```python
from build123d import *

# Parameters (mm, degrees)
BOSS_EXTRUDE1_DEPTH           = 10
BOSS_EXTRUDE1_DEPTH_BACK      = 10
SKETCH1_W                     = 11
SKETCH1_H                     = 11
SKETCH3_R                     = 1.65
M4_THREADED_3_3_MM_THRU_DEPTH = 38.199596772
CUT_EXTRUDE1_DEPTH            = 4.3
CUT_EXTRUDE1_DEPTH_BACK       = 4.3
SKETCH4_R                     = 25.3


with BuildPart() as part:
    # Sketch1 → Boss-Extrude1 (new, two sides: drawn at the far end of the back side and taken through both)
    with BuildSketch(Plane(origin=(0, 0, 0), x_dir=(0, 0, -1), z_dir=(1, 0, 0)).offset(-BOSS_EXTRUDE1_DEPTH_BACK)):
        with Locations((0, -28.6)):
            Rectangle(SKETCH1_W, SKETCH1_H)
    extrude(amount=BOSS_EXTRUDE1_DEPTH + BOSS_EXTRUDE1_DEPTH_BACK)

    # Sketch3 → M4 threaded 3.3 mm-thru (cut, through all)
    with BuildSketch(Plane.XY.offset(5.5)):
        with Locations((6, -28.6)):
            Circle(SKETCH3_R)
        with Locations((-6, -28.6)):
            Circle(SKETCH3_R)
    extrude(amount=-M4_THREADED_3_3_MM_THRU_DEPTH, mode=Mode.SUBTRACT)

    # Sketch4 → Cut-Extrude1 (cut, two sides: drawn at the far end of the back side and taken through both)
    with BuildSketch(Plane.XY.offset(-CUT_EXTRUDE1_DEPTH_BACK)):
        Circle(SKETCH4_R)
    extrude(amount=CUT_EXTRUDE1_DEPTH + CUT_EXTRUDE1_DEPTH_BACK, mode=Mode.SUBTRACT)


solid = part.part
```
Check sheet for the modelled part. Datum: model origin and axes. Units: mm. A direction names the side the tool comes from. Round coordinates to 2 decimals unless told otherwise and drop trailing zeros. Order: outer loops, then holes, each group sorted by start corner. A loop starts at its lowest first (then second) coordinate and runs counter-clockwise, first axis right, second up. Notation, with made-up numbers: (12.5, -24) - (50.5, -24) arc R32 ccw to (50.5, 9) - close; hole circle Ø8 at (6, -23.5). An arc over 180 degrees is marked (long way). Write item = value, one per line.
Q1. Go/stop test with flat-tipped pins: pin 1 (6 mm diameter, centred on x = 3.5, z = -2, fed in from +Y); pin 2 (6 mm diameter, centred on x = 5.5, z = 1, fed in from +Y). Record where each tip stops, or that it passes through.
Computed:
pin_1 = -23.1
pin_2 = -23.83
Q2. Thickness scan on line 1 along Z through (x, y) = (-8, -23.75); line 2 along Y through (x, z) = (-5.25, 5.25); line 3 along Y through (x, z) = (-6, -1). Record the ranges inside material, lowest first.
Computed:
line_1 = -5.5 to -4.3, 4.3 to 5.5
line_2 = -34.1 to -30.07, -27.13 to -23.1
line_3 = -34.1 to -30.25, -26.95 to -24.58
Q3. Draft check along Y on faces 3 (the face through (5.785, -26.964, 0.077)), 4 (the face through (-6.215, -26.964, 0.077)), 5 (the face through (10, -29, 0)), 6 (the face through (0, -34.1, 0)). Enter one of: pulls with the +Y half, pulls with the -Y half, needs draft (parallel to the pull), parting line crosses it, or undercut.
Computed:
face_3 = undercut
face_4 = undercut
face_5 = needs draft
face_6 = pulls with the -Y half
Q4. Section check B-B (x = 0). Record the boundary of the cut face in (y, z), and give its area (3 significant figures).
Computed:
outline = (-34.1, -5.5) - (-23.1, -5.5) - (-23.1, -4.3) - (-25.3, -4.3) - (-25.3, 4.3) - (-23.1, 4.3) - (-23.1, 5.5) - (-34.1, 5.5) - close
area = 102 mm^2
Q5. Section check A-A (y = -28.6). Record the boundary of the cut face in (x, z).
Computed:
outline = (-10, -5.5) - (-7.65, -5.5) - (-7.65, 5.5) - (-10, 5.5) - close; (-4.35, -5.5) - (4.35, -5.5) - (4.35, 5.5) - (-4.35, 5.5) - close; (7.65, -5.5) - (10, -5.5) - (10, 5.5) - (7.65, 5.5) - close
Q6. Section check D-D (x = 6). Record the boundary of the cut face in (y, z).
Computed:
outline = (-34.1, -5.5) - (-30.25, -5.5) - (-30.25, 5.5) - (-34.1, 5.5) - close; (-26.95, -5.5) - (-23.1, -5.5) - (-23.1, -4.3) - (-24.58, -4.3) - (-24.58, 4.3) - (-23.1, 4.3) - (-23.1, 5.5) - (-26.95, 5.5) - close
Q7. Section check C-C (z = -1.5). Record the boundary of the cut face in (x, y), and give its area (3 significant figures).
Computed:
outline = (-10, -34.1) - (10, -34.1) - (10, -23.24) arc R25.3 cw to (-10, -23.24) - close; hole circle Ø3.3 at (-6, -28.6); hole circle Ø3.3 at (6, -28.6)
area = 172 mm^2
Q8. Tool access check on faces 1 (the face through (-0.1, -25.3, -0.1)), 2 (the face through (0, -29, -5.5)). Record the directions out of +Z, -Z, +X, -X, +Y, -Y that give a thin tool (end or side, any length) a straight path to the whole face; none if there is none.
Computed:
face_1 = +Y
face_2 = -Z, +X, -X, +Y, -Y
